Autodesk Inventor part; units mm, degrees
ref_plane "YZ Plane" through (0, 0, 0) normal (1, 0, 0) x (0, 1, 0)
ref_plane "XZ Plane" through (0, 0, 0) normal (0, 1, 0) x (-1, 0, 0)
ref_plane "XY Plane" through (0, 0, 0) normal (0, 0, 1) x (1, 0, 0)
sketch "Sketch1" plane through (0, 0, 0) normal (0, 0, 1) x (1, 0, 0)
  line L0 (0, 7.3323) -> (6.35, 3.6662)
  line L1 (6.35, 3.6662) -> (6.35, -3.6662)
  line L2 (6.35, -3.6662) -> (0, -7.3323)
  line L3 (0, -7.3323) -> (-6.35, -3.6662)
  line L4 (-6.35, -3.6662) -> (-6.35, 3.6662)
  line L5 (-6.35, 3.6662) -> (0, 7.3323)
  point P0 (0, 0)
  point P1 (0, 0)
  dimension "d1" = 12.7
extrude "Extrusion1" add sketch "Sketch1" along normal mid plane 664.8247
sketch "Sketch2" plane through (0, 0, 332.4123) normal (0, 0, 1) x (1, 0, 0)
  point P0 (0, 0)
hole "Hole1" at (0, 0, 332.4123) direction (0, 0, -1) diameter 4.9784 depth 19.05 tip angle 118
mirror "Mirror1" about plane through (0, 0, 0) normal (0, 0, 1) of "Hole1"
properties part number "0.5_Jack_Shaft" material "Aluminum, 6061-T6"
Design review of the part built by this model. Coordinates are the model's own, in mm. Give positions to 0.01 mm unless a question says otherwise; leave off trailing zeros. Write each loop counter-clockwise with the first axis right and the second up, starting at its lowest first coordinate (ties: lowest second). Pieces come first, ordered by that corner, then holes. Notation, with made-up numbers: M 32,74.25 L 65,74.25 A14 cw 65,78.25 Z; hole C 60.25,0 d5. An arc over 180 degrees is marked long. Return JSON: item names as keys, results as strings. Group by question number.
Item 1: Take a section at A-A (z = -209). Give the boundary of the cut face in (x, y), plus the area to 3 significant figures.
Item 2: Wall thickness on line 1 along X through (y, z) = (0, 318); line 2 along Y through (x, z) = (0, 320.5); line 3 along X through (y, z) = (5.25, 289.5): over which ranges is each line inside the solid? List them lowest first.
Item 3: Clearance check with flat-ended pins moving along their axes: pin 1 Ø6 at (y, z) = (-4.5, -172.5) entering from +X; pin 2 Ø4 at (x, y) = (0, 0) entering from +Z; pin 3 Ø2 at (y, z) = (5, -28.5) entering from +X. State where each tip first meets the part, or that it passes through.
Return value:
{
 "1": {"outline": "M -6.35,-3.67 L 0,-7.33 L 6.35,-3.67 L 6.35,3.67 L 0,7.33 L -6.35,3.67 Z", "area": "140 mm2"},
 "2": {"line 1": "x = -6.35 to -2.49, 2.49 to 6.35", "line 2": "y = -7.33 to -2.49, 2.49 to 7.33", "line 3": "x = -3.61 to 3.61"},
 "3": {"pin 1": "stops at x = 6.35", "pin 2": "stops at z = 313.07", "pin 3": "stops at x = 5.77"}
}
